Autodesk Inventor part; units mm, degrees
ref_plane "YZ Plane" through (0, 0, 0) normal (1, 0, 0) x (0, 1, 0)
ref_plane "XZ Plane" through (0, 0, 0) normal (0, 1, 0) x (-1, 0, 0)
ref_plane "XY Plane" through (0, 0, 0) normal (0, 0, 1) x (1, 0, 0)
sketch "Skizze14" plane through (0, 0, 0) normal (0, 1, 0) x (-1, 0, 0)
  line L0 (0, 0) -> (28, 0)
  line L1 (28, 0) -> (28, 67)
  line L2 (28, 67) -> (0, 67)
  line L3 (0, 67) -> (0, 0)
  dimension "d40" = 28
  dimension "d41" = 67
extrude "Extrusion13" add sketch "Skizze14" along normal blind 10
sketch "Skizze15" plane through (-28, 0, 67) normal (0, 0, 1) x (1, 0, 0)
  line L0 (2, 8) -> (15, 8)
  line L1 (15, 8) -> (15, 2)
  line L2 (15, 2) -> (2, 2)
  line L3 (2, 2) -> (2, 8)
  dimension "d44" = 13
  dimension "d45" = 6
extrude "Extrusion14" cut sketch "Skizze15" against normal blind 13
sketch "Skizze16" plane through (-28, 0, 54) normal (0, 0, 1) x (1, 0, 0)
  line L0 (3, 8) -> (14, 8)
  line L1 (14, 8) -> (14, 3)
  line L2 (14, 3) -> (3, 3)
  line L3 (3, 3) -> (3, 8)
  point P0 (28, 0)
extrude "Extrusion15" cut sketch "Skizze16" against normal blind 60
sketch "Skizze21" plane through (0, 0, 0) normal (0, 0, -1) x (-1, 0, 0)
  line L0 (25, 8) -> (25, 3)
  line L1 (25, 3) -> (14, 3)
  line L2 (14, 3) -> (14, 8)
  line L3 (14, 8) -> (25, 8)
  line L4 (0, 0) -> (28, 0)
  line L5 (28, 0) -> (28, 10)
  line L6 (28, 10) -> (0, 10)
  line L7 (0, 10) -> (0, 0)
  line L8 (0, 0) -> (28, 0)
  line L9 (28, 0) -> (28, 10)
extrude "Extrusion20" cut sketch "Skizze21" against normal blind 17
sketch "Skizze23" plane through (-28, 0, 67) normal (0, 0, 1) x (1, 0, 0)
  line L0 (28, 0) -> (28, 10)
  line L1 (28, 0) -> (22, 0)
  line L2 (22, 0) -> (22, 10)
  line L3 (22, 10) -> (28, 10)
  line L4 (28, 10) -> (28, 0)
extrude "Extrusion22" cut sketch "Skizze23" against normal blind 60
sketch "Skizze24" plane through (0, 0, 0) normal (0, -1, 0) x (1, 0, 0)
  line L0 (-6, 17) -> (-6, 67)
  line L1 (-10, 26) -> (-6, 26)
  line L2 (-6, 26) -> (-6, 58)
  line L3 (-6, 58) -> (-10, 58)
  line L4 (-10, 58) -> (-10, 26)
  point P0 (0, 0)
extrude "Extrusion23" add sketch "Skizze24" along normal blind 8
sketch "Skizze25" plane through (-10, 0, 26) normal (-1, 0, 0) x (0, 0, 1)
  line L0 (0, 0) -> (0, -8)
  line L1 (7, -4) -> (28, -4) construction
  line L2 (7, -5.75) -> (28, -5.75)
  line L3 (28, -2.25) -> (7, -2.25)
  arc A0 (7, -2.25) -> (7, -5.75) centre (7, -4) ccw
  arc A1 (28, -5.75) -> (28, -2.25) centre (28, -4) ccw
  point P0 (-26, 0)
  point P1 (17.5, -4)
  dimension "d70" = 3.5
extrude "Extrusion24" cut sketch "Skizze25" against normal blind 12
sketch "Skizze26" plane through (-10, 0, 26) normal (-1, 0, 0) x (0, 0, 1)
  arc A0 (28, -5.75) -> (28, -2.25) centre (28, -4) ccw
  line L0 (28, -5.75) -> (7, -5.75)
  arc A1 (7, -2.25) -> (7, -5.75) centre (7, -4) ccw
  line L1 (7, -2.25) -> (28, -2.25)
  line L2 (0, 0) -> (32, 0)
  line L3 (0, 0) -> (0, -8)
  line L4 (32, -8) -> (0, -8)
  line L5 (32, 0) -> (32, -8)
  point P0 (-26, 0)
properties part number "OPB732_CASE_BOTTOM"
Could you check a few things on this model? Use its own coordinates, in mm. A direction names the side the tool comes from. Coordinates: 2 decimals unless noted, no trailing zeros. Loops run counter-clockwise (first coordinate to the right, second up) from the corner with the lowest first, then second, coordinate; pieces in that order, holes last.
1) Imagine slicing it at C-C (y = -4). List the corners of the cut face in (x, z) for me.
Reported:
outline: (-10, 26) - (-6, 26) - (-6, 31.25) - (-10, 31.25) - close; (-10, 55.75) - (-6, 55.75) - (-6, 58) - (-10, 58) - close
2) Will these pins go through, and if not, where does the flat tip stop? pin 1 Ø4 at (y, z) = (-4.5, 35.5) entering from -X; pin 2 Ø6 at (x, y) = (-17, 3.5) entering from +Z; pin 3 Ø5 at (x, z) = (-22, 49.5) entering from -Y; pin 4 Ø2 at (x, y) = (-8, -3) entering from +Z.
Reported:
pin 1: stops at x = -10
pin 2: stops at z = 67
pin 3: stops at y = 0
pin 4: stops at z = 58
3) Imagine slicing it at A-A (z = 45). List the corners of the cut face in (x, y) for me.
Reported:
outline: (-28, 0) - (-10, 0) - (-10, -2.25) - (-6, -2.25) - (-6, 10) - (-28, 10) - close; (-10, -8) - (-6, -8) - (-6, -5.75) - (-10, -5.75) - close; hole (-25, 3) - (-14, 3) - (-14, 8) - (-25, 8) - close
4) Imagine slicing it at B-B (x = -16.75). List the corners of the cut face in (y, z) for me.
Reported:
outline: (0, 17) - (3, 17) - (3, 54) - (2, 54) - (2, 67) - (0, 67) - close; (8, 17) - (10, 17) - (10, 67) - (8, 67) - close
5) Imagine slicing it at D-D (y = 2.5). List the corners of the cut face in (x, z) for me, and give its area (3 significant figures).
Reported:
outline: (-28, 17) - (-6, 17) - (-6, 67) - (-13, 67) - (-13, 54) - (-26, 54) - (-26, 67) - (-28, 67) - close
area: 931 mm2
6) Please list where these lines run through material, in increasing order: line 1 along Y through (x, z) = (-9.5, 41); line 2 along X through (y, z) = (3.5, 58.5); line 3 along Y through (x, z) = (-18.5, 27).
Reported:
line 1: y = -8 to -5.75, -2.25 to 10
line 2: x = -28 to -26, -13 to -6
line 3: y = 0 to 3, 8 to 10
7) Thinking about a two-plate mould opening in Z: for faces 1 (the face through (-17, 0, 42)), 2 (the face through (-16.8, 2.8, 17)), 3 (the face through (-8.03, -4.04, 55.75)), which applies, released by +Z, released by -Z, zero draft, split by the parting line, or undercut?
Reported:
face 1: zero draft
face 2: released by -Z
face 3: undercut
8) Which directions (+Z, -Z, +X, -X, +Y, -Y) give clear straight access to the entire face, cutting with the end or side of a thin tool? Please do faces 4 (the face through (-8.03, -3.96, 31.25)), 5 (the face through (-10, -2, 42)), 6 (the face through (-26, 5, 61)), 7 (the face through (-14, 6, 36)).
Reported:
face 4: +X, -X
face 5: +Z, -Z, -X, -Y
face 6: +Z
face 7: +Z, -Z
